```python
from build123d import *

# Parameters (mm, degrees)
SKETCH2_W               = 103
SKETCH2_H               = 65
BOSS_EXTRUDE1_DEPTH     = 9.8
SKETCH4_W               = 97
SKETCH4_H               = 40
CUT_EXTRUDE1_DEPTH      = 35
SKETCH6_W               = 42.890315644
SKETCH6_H               = 9.943201627
CUT_EXTRUDE3_DEPTH      = 6
SKETCH9_W               = 103
SKETCH9_H               = 65
SKETCH9_W_2             = 98
SKETCH9_H_2             = 60
BOSS_EXTRUDE2_DEPTH     = 1.6
SKETCH10_W              = 42.890315644
SKETCH10_H              = 16.344193147
CUT_EXTRUDE4_DEPTH      = 9.943201627
CUT_EXTRUDE7_DEPTH      = 28
CUT_EXTRUDE7_DEPTH_BACK = 33
SKETCH14_R              = 1.629970135
SKETCH14_R_2            = 1.938580121
SKETCH14_R_3            = 1.388390768
SKETCH14_R_4            = 1.438089521


with BuildPart() as part:
    # Sketch2 → Boss-Extrude1 (new body)
    with BuildSketch(Plane.XY):
        Rectangle(SKETCH2_W, SKETCH2_H)
    extrude(amount=BOSS_EXTRUDE1_DEPTH)

    # Sketch4 → Cut-Extrude1 (cut)
    with BuildSketch(Plane.XY.offset(9.8)):
        Rectangle(SKETCH4_W, SKETCH4_H)
    extrude(amount=-CUT_EXTRUDE1_DEPTH, mode=Mode.SUBTRACT)

    # Sketch6 → Cut-Extrude3 (cut)
    with BuildSketch(Plane(origin=(0, 0, 0), x_dir=(-1, 0, 0), z_dir=(0, 0, -1))):
        with Locations((20.148258429, 27.528399187)):
            Rectangle(SKETCH6_W, SKETCH6_H)
    extrude(amount=-CUT_EXTRUDE3_DEPTH, mode=Mode.SUBTRACT)

    # Sketch9 → Boss-Extrude2 (add)
    with BuildSketch(Plane(origin=(0, 0, 0), x_dir=(-1, 0, 0), z_dir=(0, 0, -1))):
        Rectangle(SKETCH9_W, SKETCH9_H)
        Rectangle(SKETCH9_W_2, SKETCH9_H_2, mode=Mode.SUBTRACT)
    extrude(amount=BOSS_EXTRUDE2_DEPTH)

    # Sketch10 → Cut-Extrude4 (cut)
    with BuildSketch(Plane(origin=(0, 32.5, 0), x_dir=(1, 0, 0), z_dir=(0, 1, 0))):
        with Locations((-20.148258429, 8.172096574)):
            Rectangle(SKETCH10_W, SKETCH10_H)
    extrude(amount=-CUT_EXTRUDE4_DEPTH, mode=Mode.SUBTRACT)

    # Sketch14 → Cut-Extrude7 (cut, two sides: drawn at the far end of the back side and taken through both)
    with BuildSketch(Plane(origin=(0, 0, -1.6), x_dir=(-1, 0, 0), z_dir=(0, 0, -1)).offset(-CUT_EXTRUDE7_DEPTH_BACK)):
        with Locations((-46.5, 27.5)):
            Circle(SKETCH14_R)
        with Locations((46.5, 27.5)):
            Circle(SKETCH14_R_2)
        with Locations((46.5, -27.5)):
            Circle(SKETCH14_R_3)
        with Locations((-46.5, -27.5)):
            Circle(SKETCH14_R_4)
    extrude(amount=CUT_EXTRUDE7_DEPTH + CUT_EXTRUDE7_DEPTH_BACK, mode=Mode.SUBTRACT)


solid = part.part
```
Geometry check sheet. Reference: the model listing, model coordinates, mm. A direction names the side the tool comes from. Coordinates: 2 decimals unless noted, no trailing zeros. Order: outer loops, then holes, each group sorted by start corner. A loop starts at its lowest first (then second) coordinate and runs counter-clockwise, first axis right, second up. Notation, with made-up numbers: (70.25, 45) - (84.25, 45) arc R19 ccw to (84.25, 68) - close; hole circle Ø8 at (-9.5, 25.5). An arc over 180 degrees is marked (long way). Answer in a Markdown table with one row per item. Add a question column.
1. Material ranges on L1, parallel to Y at x = 46.5, z = 4.5; L2, parallel to X at y = -27.5, z = 2.75; L3, parallel to Y at x = -46.5, z = 6.5, recorded low to high. Write a range as [from, to].
2. Section check B-B (x = 46.5). Enter the section's corners in (y, z).
3. Draft check along Y on faces 1 (the face through (-1, 22, 9.8)), 2 (the face through (12, 32.5, 5)), 3 (the face through (48.5, 0, 5)), 4 (the face through (45.748, 26.054, 4.969)). Enter one of: +Y half, -Y half, draft (parallel to the pull), parting line (faces both ways), or undercut.
4. Section check C-C (y = -11). Enter the section's corners in (x, z).
5. Section check A-A (y = -27.5). Enter the section's corners in (x, z).
6. Gauge pin test, flat ends, axial feed: pin 1 Ø2.5 at (x, y) = (-46.5, 27.5) entering from +Z; pin 2 Ø5 at (x, y) = (46.5, 27.5) entering from +Z; pin 3 Ø3 at (x, y) = (-21.5, 26.5) entering from -Z; pin 4 Ø1.8 at (x, z) = (-26, 1.5) entering from +Y. Record the tip position at first contact, or that the pin passes through.
7. Section check D-D (x = -17). Enter the section's corners in (y, z).
8. Access from +Z, -Z, +X, -X, +Y, -Y to the whole of each face (thin tool, end or side, straight path). Record for faces 5 (the face through (-4, 22, 0)), 6 (the face through (-51.5, 0, 4)), 7 (the face through (-20, 28, 6)), 8 (the face through (-1, -20, 5)), 9 (the face through (4, -31, -1.6)).
Data:
| question | item | result |
|---|---|---|
| 1 | L1 | y = [-32.5, -28.94], [-26.06, -20], [20, 25.87], [29.13, 32.5] |
| 1 | L2 | x = [-51.5, -47.89], [-45.11, 45.06], [47.94, 51.5] |
| 1 | L3 | y = [-32.5, -28.89], [-26.11, -20], [20, 25.56], [29.44, 32.5] |
| 2 | outline | (-32.5, -1.6) - (-30, -1.6) - (-30, 0) - (-28.94, 0) - (-28.94, 9.8) - (-32.5, 9.8) - close; (-26.06, 0) - (-20, 0) - (-20, 9.8) - (-26.06, 9.8) - close; (20, 0) - (25.87, 0) - (25.87, 9.8) - (20, 9.8) - close; (29.13, 0) - (30, 0) - (30, -1.6) - (32.5, -1.6) - (32.5, 9.8) - (29.13, 9.8) - close |
| 3 | face 1 | draft |
| 3 | face 2 | +Y half |
| 3 | face 3 | undercut |
| 3 | face 4 | undercut |
| 4 | outline | (-51.5, -1.6) - (-49, -1.6) - (-49, 0) - (-48.5, 0) - (-48.5, 9.8) - (-51.5, 9.8) - close; (48.5, 0) - (49, 0) - (49, -1.6) - (51.5, -1.6) - (51.5, 9.8) - (48.5, 9.8) - close |
| 5 | outline | (-51.5, -1.6) - (-49, -1.6) - (-49, 0) - (-47.89, 0) - (-47.89, 9.8) - (-51.5, 9.8) - close; (-45.11, 0) - (45.06, 0) - (45.06, 9.8) - (-45.11, 9.8) - close; (47.94, 0) - (49, 0) - (49, -1.6) - (51.5, -1.6) - (51.5, 9.8) - (47.94, 9.8) - close |
| 6 | pin 1 | passes through |
| 6 | pin 2 | stops at z = 9.8 |
| 6 | pin 3 | stops at z = 6 |
| 6 | pin 4 | stops at y = 22.56 |
| 7 | outline | (-32.5, -1.6) - (-30, -1.6) - (-30, 0) - (-20, 0) - (-20, 9.8) - (-32.5, 9.8) - close; (20, 0) - (22.56, 0) - (22.56, 6) - (32.5, 6) - (32.5, 9.8) - (20, 9.8) - close |
| 8 | face 5 | -Z |
| 8 | face 6 | +Z, -Z, -X, +Y, -Y |
| 8 | face 7 | -Z, +Y |
| 8 | face 8 | +Z, -Z |
| 8 | face 9 | -Z, +X, -X, +Y, -Y |
